Geometry: final body of the model. Coordinates: model frame, mm. A direction names the side the tool comes from. Give positions to 0.01 mm unless a question says otherwise; leave off trailing zeros. Order: outer loops, then holes, each group sorted by start corner. A loop starts at its lowest first (then second) coordinate and runs counter-clockwise, first axis right, second up. Notation, with made-up numbers: (-3.75, -17.5) -> (35.25, -17.5) arc R17 cw to (35.25, -7.5) -> close; hole circle Ø1 at (21.25, 2). An arc over 180 degrees is marked (long way). One line per question, with ' | ' between items. Start each with the question number.
(1) First-contact query: pin 1 Ø2 at (y, z) = (124, 120.5) entering from +X. Flat tip, straight axial feed; report the tip coordinate or a pass-through.
(2) Set-up query: faces 1 (the face through (75, 194, 111)), 2 (the face through (47, 12, 111)). Return all of +Z, -Z, +X, -X, +Y, -Y with unobstructed straight access to the full face (end or side cutting, diameter ignored); none if empty.
(3) Section B-B (x = 33.5). Return loops of the section in (y, z).
(4) Section A-A (z = 45). Return loops of the section in (x, y).
(5) Ray query, L1, parallel to Z at x = 1.65, y = 100; L2, parallel to Y at x = 29, z = 183.5; L3, parallel to Y at x = 2, z = 45. Return the intervals inside material, ascending.
(6) Section D-D (x = 15). Return loops of the section in (y, z), then the cut area to 3 significant figures.
(7) Section C-C (y = 100). Return loops of the section in (x, z), then the cut area to 3 significant figures.
(8) Mould query, pull axis Y, two halves, no side actions, for faces 3 (the face through (38, 200, 111)), 4 (the face through (4, 100, 225)), 5 (the face through (9.61, 15.42, 110.92)). Classes: +Y half, -Y half, draft (parallel to the pull), parting line (faces both ways), or undercut.
```python
from build123d import *

# Parameters (mm, degrees)
F1_DEPTH = 225
F2_R     = 5.5
F3_DEPTH = 75.001


with BuildPart() as f1:
    # F0 (on Top) → F1 (new body)
    with BuildSketch(Plane.XY):
        with BuildLine():
            Line((0, 200), (0, 0))
            Line((0, 0), (75, 0))
            Line((75, 0), (75, 12))
            Line((75, 12), (18, 12))
            ThreePointArc((18, 12), (9.514719, 15.514719), (6, 24))
            Line((6, 24), (6, 176))
            ThreePointArc((6, 176), (9.514719, 184.485281), (18, 188))
            Line((18, 188), (75, 188))
            Line((75, 188), (75, 200))
            Line((75, 200), (0, 200))
        make_face()
    extrude(amount=F1_DEPTH)

    # F2 (on Right) → F3 (cut, through all)
    with BuildSketch(Plane.YZ):
        with Locations((100, 195)):
            Circle(F2_R)
        with Locations((100, 45)):
            Circle(F2_R)
    extrude(amount=F3_DEPTH, mode=Mode.SUBTRACT)


solid = f1.part
```
Response:
1) pin 1: stops at x = 6
2) face 1: +Z, -Z, +X, +Y, -Y | face 2: +Z, -Z, +X
3) outline: (0, 0) -> (12, 0) -> (12, 225) -> (0, 225) -> close; (188, 0) -> (200, 0) -> (200, 225) -> (188, 225) -> close
4) outline: (0, 0) -> (75, 0) -> (75, 12) -> (18, 12) arc R12 cw to (6, 24) -> (6, 94.5) -> (0, 94.5) -> close; (0, 105.5) -> (6, 105.5) -> (6, 176) arc R12 cw to (18, 188) -> (75, 188) -> (75, 200) -> (0, 200) -> close
5) L1: z = 0 to 39.5, 50.5 to 189.5, 200.5 to 225 | L2: y = 0 to 12, 188 to 200 | L3: y = 0 to 94.5, 105.5 to 200
6) outline: (0, 0) -> (12.38, 0) -> (12.38, 225) -> (0, 225) -> close; (187.62, 0) -> (200, 0) -> (200, 225) -> (187.62, 225) -> close | area: 5,570 mm^2
7) outline: (0, 0) -> (6, 0) -> (6, 39.5) -> (0, 39.5) -> close; (0, 50.5) -> (6, 50.5) -> (6, 189.5) -> (0, 189.5) -> close; (0, 200.5) -> (6, 200.5) -> (6, 225) -> (0, 225) -> close | area: 1,220 mm^2
8) face 3: +Y half | face 4: draft | face 5: undercut
